from build123d import *

# Parameters (mm, degrees)
SKETCH_1_W          = 53
SKETCH_1_H          = 40
EXTRUDE_1_DEPTH     = 24.2
CUT_EXTRUDE_1_DEPTH = 71.672767032
SKETCH_3_R          = 1.5
CUT_EXTRUDE_2_DEPTH = 71.672767032


with BuildPart() as part:
    # 草图1 → 凸台-拉伸1 (new body)
    with BuildSketch(Plane.XY):
        with Locations((26.5, 20)):
            Rectangle(SKETCH_1_W, SKETCH_1_H)
    extrude(amount=EXTRUDE_1_DEPTH)

    # 草图2 → 切除-拉伸1 (cut, through all)
    with BuildSketch(Plane.XY.offset(24.2)):
        Polygon((53, 28), (53, 0), (25, 0), align=None)
    extrude(amount=-CUT_EXTRUDE_1_DEPTH, mode=Mode.SUBTRACT)

    # 草图3 → 切除-拉伸2 (cut, through all)
    with BuildSketch(Plane.XY.offset(24.2)):
        with Locations((5, 30)):
            Circle(SKETCH_3_R)
        with Locations((5, 6)):
            Circle(SKETCH_3_R)
        with Locations((22, 30)):
            Circle(SKETCH_3_R)
        with Locations((22, 6)):
            Circle(SKETCH_3_R)
        with Locations((42, 30)):
            Circle(SKETCH_3_R)
    extrude(amount=-CUT_EXTRUDE_2_DEPTH, mode=Mode.SUBTRACT)


solid = part.part
Could you check a few things on this model? Use its own coordinates, in mm. Coordinates: 2 decimals unless noted, no trailing zeros. Loops run counter-clockwise (first coordinate to the right, second up) from the corner with the lowest first, then second, coordinate; pieces in that order, holes last. Notation, with made-up numbers: (42, -12.5) -> (52, -12.5) arc R26 cw to (52, 18.5) -> close; hole circle Ø7 at (62, 67.25). An arc over 180 degrees is marked (long way). Answer in a Markdown table with one row per item.
(1) If I drill on probe 1 along Y at (x, z) = (5, 9.25); probe 2 along X at (y, z) = (31, 13.5); probe 3 along Y at (x, z) = (42, 15), over which ranges is the centre line in solid material (lowest first)?
Results found:
| item | result |
|---|---|
| probe 1 | y = 0 to 4.5, 7.5 to 28.5, 31.5 to 40 |
| probe 2 | x = 0 to 3.88, 6.12 to 20.88, 23.12 to 40.88, 43.12 to 53 |
| probe 3 | y = 17 to 28.5, 31.5 to 40 |
(2) Imagine slicing it at D-D (z = 13.25). List the corners of the cut face in (x, y) for me.
Results found:
| item | result |
|---|---|
| outline | (0, 0) -> (25, 0) -> (53, 28) -> (53, 40) -> (0, 40) -> close; hole circle Ø3 at (5, 6); hole circle Ø3 at (5, 30); hole circle Ø3 at (22, 6); hole circle Ø3 at (22, 30); hole circle Ø3 at (42, 30) |
(3) Imagine slicing it at A-A (y = 6). List the corners of the cut face in (x, z) for me, plus the area to 3 significant figures.
Results found:
| item | result |
|---|---|
| outline | (0, 0) -> (3.5, 0) -> (3.5, 24.2) -> (0, 24.2) -> close; (6.5, 0) -> (20.5, 0) -> (20.5, 24.2) -> (6.5, 24.2) -> close; (23.5, 0) -> (31, 0) -> (31, 24.2) -> (23.5, 24.2) -> close |
| area | 605 mm^2 |
(4) Thinking about a two-plate mould opening in Y: for faces 1 (the face through (20, 25, 24.2)), 2 (the face through (4.805, 31.487, 12.269)), 3 (the face through (12, 0, 12)), which applies, released by +Y, released by -Y, zero draft, split by the parting line, or undercut?
Results found:
| item | result |
|---|---|
| face 1 | zero draft |
| face 2 | undercut |
| face 3 | released by -Y |
(5) Imagine slicing it at B-B (x = 22). List the corners of the cut face in (y, z) for me.
Results found:
| item | result |
|---|---|
| outline | (0, 0) -> (4.5, 0) -> (4.5, 24.2) -> (0, 24.2) -> close; (7.5, 0) -> (28.5, 0) -> (28.5, 24.2) -> (7.5, 24.2) -> close; (31.5, 0) -> (40, 0) -> (40, 24.2) -> (31.5, 24.2) -> close |
(6) Imagine slicing it at C-C (x = 42). List the corners of the cut face in (y, z) for me, plus the area to 3 significant figures.
Results found:
| item | result |
|---|---|
| outline | (17, 0) -> (28.5, 0) -> (28.5, 24.2) -> (17, 24.2) -> close; (31.5, 0) -> (40, 0) -> (40, 24.2) -> (31.5, 24.2) -> close |
| area | 484 mm^2 |
(7) Will these pins go through, and if not, where does the flat tip stop? pin 1 Ø1.5 at (y, z) = (23.5, 17) entering from +X; pin 2 Ø2 at (y, z) = (17.5, 5.5) entering from +X.
Results found:
| item | result |
|---|---|
| pin 1 | stops at x = 49.25 |
| pin 2 | stops at x = 43.5 |
